Verification items for the finished model (mm, model axes). Face numbers are marked on the shaded views. A direction names the side the tool comes from. Give positions to 0.01 mm unless a question says otherwise; leave off trailing zeros. Order: outer loops, then holes, each group sorted by start corner. A loop starts at its lowest first (then second) coordinate and runs counter-clockwise, first axis right, second up.
(1) Sectioned sample at B-B on x = 0. Record the cut outline in (y, z).
(2) Scan lines: L1, parallel to X at y = 12, z = 5; L2, parallel to X at y = -9.95, z = 5; L3, parallel to Y at x = 0, z = 1.5. Record each from-to range of solid material in increasing order.
(3) Sectioned sample at A-A on y = -1.5. Record the cut outline in (x, z).
(4) Sectioned sample at D-D on z = 3.5. Record the cut outline in (x, y), plus the area to 3 significant figures.
(5) Access from +Z, -Z, +X, -X, +Y, -Y to the whole of each face (thin tool, end or side, straight path). Record for the marked faces 1, 2 and 3.
(6) Mould release check, pull along Z, two halves, no side actions. Record for the marked faces 4, 5 and 6: pulls with the +Z half, pulls with the -Z half, needs draft (parallel to the pull), parting line crosses it, or undercut.
(7) Gauge pin test, flat ends, axial feed: pin 1 (3.5 mm diameter, centred on x = -11.5, z = 4.5, fed in from -Y); pin 2 (13 mm diameter, centred on x = 0, y = -1.5, fed in from +Z); pin 3 (10.5 mm diameter, centred on x = 0, y = -1.5, fed in from -Z). Record the tip position at first contact, or that the pin passes through.
(8) Sectioned sample at C-C on x = -11. Record the cut outline in (y, z), plus the area to 3 significant figures.
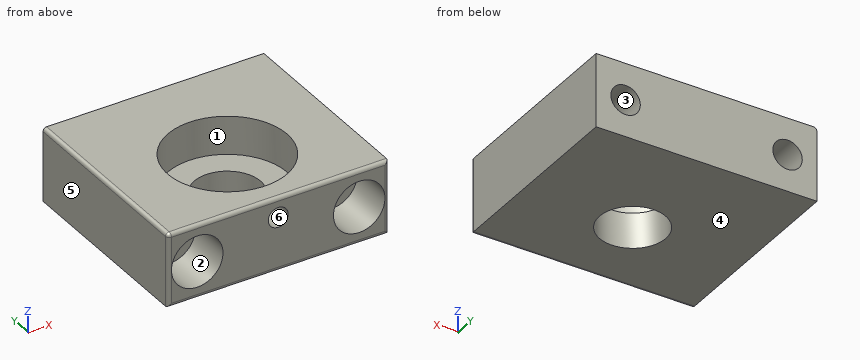
Autodesk Inventor part; units mm, degrees
ref_plane "YZ Plane" through (0, 0, 0) normal (1, 0, 0) x (0, 1, 0)
ref_plane "XZ Plane" through (0, 0, 0) normal (0, 1, 0) x (-1, 0, 0)
ref_plane "XY Plane" through (0, 0, 0) normal (0, 0, 1) x (1, 0, 0)
sketch "Sketch1" plane through (0, 0, 0) normal (0, 0, 1) x (1, 0, 0)
  line L0 (-15, 12.5) -> (15, 12.5)
  line L1 (15, 12.5) -> (15, -12.5)
  line L2 (15, -12.5) -> (-15, -12.5)
  line L3 (-15, -12.5) -> (-15, 12.5)
  line L4 (-15, 12.5) -> (15, -12.5) construction
  line L5 (15, 12.5) -> (-15, -12.5) construction
  point P0 (0, 0)
  dimension "d13" = 4
  dimension "d0" = 30
  dimension "d10" = 25
extrude "Extrusion1" add sketch "Sketch1" along normal blind 10
sketch "Sketch2" plane through (0, 0, 10) normal (0, 0, 1) x (1, 0, 0)
  circle A0 centre (0, -1.5) radius 8.1
  line L0 (15, 12.5) -> (-15, 12.5)
  point P0 (0, 12.5)
  dimension "d4" = 16.2
  dimension "d38" = 14
extrude "Extrusion2" cut sketch "Sketch2" against normal blind 5.2
sketch "Sketch3" plane through (0, -1.5, 4.8) normal (0, 0, 1) x (1, 0, 0)
  circle A0 centre (0, 0) radius 4.5
  circle A1 centre (0, 0) radius 8.1
  dimension "d7" = 9
extrude "Extrusion3" cut sketch "Sketch3" against normal blind 5.2 contours A0
sketch "Sketch4" plane through (-15, -12.5, 0) normal (0, -1, 0) x (1, 0, 0)
  line L0 (0, 0) -> (0, 10)
  line L1 (0, 10) -> (30, 10)
  point P0 (15, 0)
  point P1 (4, 5)
  dimension "d11" = 4
  dimension "d12" = 5
hole "Hole1" at (-11, -12.5, 5) direction (0, 1, 0) diameter 4 end through all counterbore diameter 7 counterbore depth 6
sketch "Sketch5" plane through (-15, -12.5, 0) normal (0, -1, 0) x (1, 0, 0)
  line L0 (30, 0) -> (30, 10)
  line L1 (0, 10) -> (30, 10)
  point P0 (15, 0)
  point P1 (26, 5)
  dimension "d20" = 4
  dimension "d21" = 5
hole "Hole2" at (11, -12.5, 5) direction (0, 1, 0) diameter 4 end through all counterbore diameter 7 counterbore depth 6
sketch "Sketch6" plane through (-15, -12.5, 0) normal (0, -1, 0) x (1, 0, 0)
  line L0 (0, 10) -> (30, 10)
  line L1 (30, 0) -> (30, 10)
  point P0 (15, 0)
  point P1 (15, 7.3)
  dimension "d29" = 2.7
  dimension "d30" = 15
hole "Hole3" at (0, -12.5, 7.3) direction (0, 1, 0) diameter 2.7 depth 8 tip angle 118
fillet "Fillet2" radius 0.5 5 edges at (-15, 0, 10) (0, -12.5, 0) (15, -12.5, 5) (-15, -12.5, 5) (0, -12.5, 10)
move faces "Move1" translate (0, 2, 0) faces at (3.3569, 12.5, 1.0764)
properties part number "wheel_holder_2"
Ans:
1. outline: (-12.5, 0.5) arc R0.5 ccw to (-12, 0) - (-6, 0) - (-6, 4.8) - (-9.6, 4.8) - (-9.6, 5.95) - (-12.5, 5.95) - close; (-12.5, 8.65) - (-9.6, 8.65) - (-9.6, 10) - (-12, 10) arc R0.5 ccw to (-12.5, 9.5) - close; (3, 0) - (14.5, 0) - (14.5, 10) - (6.6, 10) - (6.6, 4.8) - (3, 4.8) - close
2. L1: x = -15 to -13, -9 to 9, 13 to 15
2. L2: x = -15 to -14.5, -7.5 to 7.5, 14.5 to 15
2. L3: y = -12.5 to -6, 3 to 14.5
3. outline: (-15, 0) - (-4.5, 0) - (-4.5, 4.8) - (-8.1, 4.8) - (-8.1, 10) - (-14.5, 10) arc R0.5 ccw to (-15, 9.5) - close; (4.5, 0) - (15, 0) - (15, 10) - (8.1, 10) - (8.1, 4.8) - (4.5, 4.8) - close; hole circle Ø4 at (-11, 5); hole circle Ø4 at (11, 5)
4. outline: (-15, -12) arc R0.5 ccw to (-14.5, -12.5) - (-14.16, -12.5) - (-14.16, -6.5) - (-12.32, -6.5) - (-12.32, 14.5) - (-15, 14.5) - close; (-9.68, -6.5) - (-7.84, -6.5) - (-7.84, -12.5) - (7.84, -12.5) - (7.84, -6.5) - (9.68, -6.5) - (9.68, 14.5) - (-9.68, 14.5) - close; (12.32, -6.5) - (14.16, -6.5) - (14.16, -12.5) - (14.5, -12.5) arc R0.5 ccw to (15, -12) - (15, 14.5) - (12.32, 14.5) - close; hole circle Ø9 at (0, -1.5)
4. area: 559 mm2
5. face 1: +Z
5. face 2: -Y
5. face 3: +Y, -Y
6. face 4: pulls with the -Z half
6. face 5: needs draft
6. face 6: undercut
7. pin 1: stops at y = -6.5
7. pin 2: stops at z = 4.8
7. pin 3: stops at z = 0
8. outline: (-12.5, 0.5) arc R0.5 ccw to (-12, 0) - (14.5, 0) - (14.5, 3) - (-6.5, 3) - (-6.5, 1.5) - (-12.5, 1.5) - close; (-12.5, 8.5) - (-6.5, 8.5) - (-6.5, 7) - (14.5, 7) - (14.5, 10) - (-12, 10) arc R0.5 ccw to (-12.5, 9.5) - close
8. area: 144 mm2
